Autodesk Inventor part; units mm, degrees
ref_plane "YZ Plane" through (0, 0, 0) normal (1, 0, 0) x (0, 1, 0)
ref_plane "XZ Plane" through (0, 0, 0) normal (0, 1, 0) x (-1, 0, 0)
ref_plane "XY Plane" through (0, 0, 0) normal (0, 0, 1) x (1, 0, 0)
sketch "Sketch1" plane through (0, 0, 0) normal (0, 0, 1) x (1, 0, 0)
  line L0 (0, 0) -> (165.1, 0)
  line L1 (165.1, 0) -> (165.1, 9.525)
  line L2 (165.1, 9.525) -> (0, 9.525)
  line L3 (0, 9.525) -> (0, 0)
  dimension "d0" = 165.1
  dimension "d1" = 9.525
extrude "Extrusion1" add sketch "Sketch1" along normal blind 3.175
sketch "Sketch2" plane through (0, 0, 3.175) normal (0, 0, 1) x (1, 0, 0)
  line L0 (165.1, 9.525) -> (0, 9.525)
  line L1 (0, 9.525) -> (0, 0)
  circle A0 centre (3.81, 4.7625) radius 0.5592
  point P0 (82.55, 4.7625)
  point P1 (161.29, 4.7625)
  dimension "d4" = 3.81
  dimension "d5" = 4.7625
  dimension "d8" = 78.74
hole "Hole1" at (3.81, 4.7625, 3.175) at (82.55, 4.7625, 3.175) at (161.29, 4.7625, 3.175) direction (0, 0, -1) diameter 4.4958 end through all
draft "FaceDraft3" angle 16 pull direction (0, 1, 0) faces at (82.55, 0.8382, 3.175) fixed edges at (82.55, 9.525, 3.175)
properties part number "bar"
Could you check a few things on this model? Use its own coordinates, in mm. Round coordinates to 2 decimals unless told otherwise and drop trailing zeros. Loops run counter-clockwise (first coordinate to the right, second up) from the corner with the lowest first, then second, coordinate; pieces in that order, holes last.
Q1. Please list where these lines run through material, in increasing order: L1, parallel to X at y = 5.25, z = 3.7; L2, parallel to X at y = 3.75, z = 3.55; L3, parallel to Z at x = 143, y = 2.5.
Q2. I want a section at C-C (x = 87). Write out the boundary of the cut face in (y, z) (3 decimals), and give its area (3 significant figures).
Q3. Thinking about a two-plate mould opening in X: for faces 1 (the flat face through (81.394, 6.946, 3.915)), 2 (the cylindrical face through (3.13, 2.62, 2.56)), 3 (the flat face through (0, 5, 2)), which applies, pulls with the +X half, pulls with the -X half, needs draft (parallel to the pull), parting line crosses it, or undercut?
Q4. I want a section at B-B (x = 3.81). Write out the boundary of the cut face in (y, z) (3 decimals).
Q5. I want a section at D-D (z = 4.1). Write out the boundary of the cut face in (x, y), and give its area (3 significant figures).
Q6. I want a section at A-A (y = 5). Write out the boundary of the cut face in (x, z).
Answer below:
1. L1: x = 0 to 1.62, 6 to 80.36, 84.74 to 159.1, 163.48 to 165.1
1. L2: x = 0 to 1.8, 5.82 to 80.54, 84.56 to 159.28, 163.3 to 165.1
1. L3: z = 0 to 5.19
2. outline: (0, 0) - (9.525, 0) - (9.525, 3.175) - (0, 5.906) - close
2. area: 43.2 mm2
3. face 1: needs draft
3. face 2: undercut
3. face 3: pulls with the -X half
4. outline: (0, 0) - (2.515, 0) - (2.515, 5.185) - (0, 5.906) - close; (7.01, 0) - (9.525, 0) - (9.525, 3.175) - (7.01, 3.896) - close
5. outline: (0, 0) - (165.1, 0) - (165.1, 6.3) - (162.93, 6.3) arc R2.25 cw (long way) to (159.65, 6.3) - (84.19, 6.3) arc R2.25 cw (long way) to (80.91, 6.3) - (5.45, 6.3) arc R2.25 cw (long way) to (2.17, 6.3) - (0, 6.3) - close
5. area: 997 mm2
6. outline: (0, 0) - (1.57, 0) - (1.57, 4.47) - (0, 4.47) - close; (6.05, 0) - (80.31, 0) - (80.31, 4.47) - (6.05, 4.47) - close; (84.79, 0) - (159.05, 0) - (159.05, 4.47) - (84.79, 4.47) - close; (163.53, 0) - (165.1, 0) - (165.1, 4.47) - (163.53, 4.47) - close
